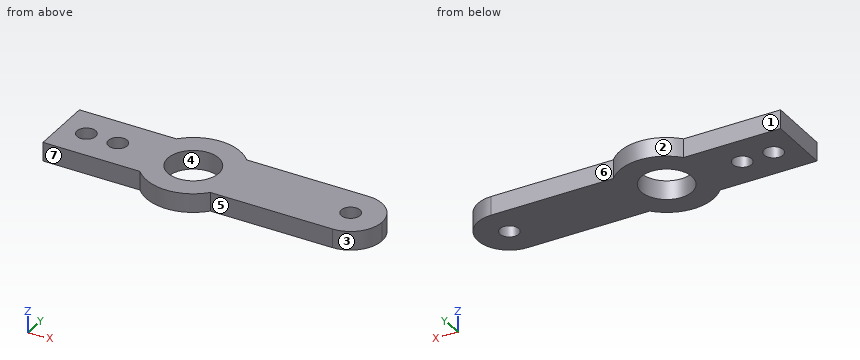
from build123d import *

# Parameters (mm, degrees)
F0_R     = 1.5
F0_R_2   = 4.05
F1_DEPTH = 3
F2_W     = 10
F2_H     = 3
F3_DEPTH = 9
F4_R     = 1.5
F5_DEPTH = 25
F6_R     = 4.99999


# Not quite as in the source:
# - a fillet or chamfer is up to 0.001 mm smaller than in the source, because OpenCascade refuses the exact size


with BuildPart() as f1:
    # F0 (on Top) → F1 (new body)
    with BuildSketch(Plane.XY):
        Polygon((21, -5), (21, 5), (5.5901699437, 5), (-5.5901699437, 5), (-21, 5), (-21, -5), (-5.5901699437, -5), (5.5901699437, -5), align=None)
        with Locations((-17, 0)):
            Circle(F0_R, mode=Mode.SUBTRACT)
        with Locations((-12, 0)):
            Circle(F0_R, mode=Mode.SUBTRACT)
        Circle(F0_R_2, mode=Mode.SUBTRACT)
        with BuildLine():
            Line((-5.5901699437, 5), (5.5901699437, 5))
            ThreePointArc((5.5901699437, 5), (0, 7.5), (-5.5901699437, 5))
        make_face()
        with BuildLine():
            ThreePointArc((-5.5901699437, -5), (0, -7.5), (5.5901699437, -5))
            Line((5.5901699437, -5), (-5.5901699437, -5))
        make_face()
    extrude(amount=F1_DEPTH)

    # F2 (on face) → F3 (join)
    with BuildSketch(Plane.YZ.offset(21)):
        with Locations((0, 1.5)):
            Rectangle(F2_W, F2_H)
    extrude(amount=F3_DEPTH)

    # F4 (on face) → F5 (cut)
    with BuildSketch(Plane(origin=(0, 0, 0), x_dir=(1, 0, 0), z_dir=(0, 0, -1))):
        with Locations((25, 0)):
            Circle(F4_R)
    extrude(amount=-F5_DEPTH, mode=Mode.SUBTRACT)

    # F6 (radius 5 in the source; OpenCascade refuses exactly that, so slightly less here)
    f6_edges = [f1.edges().sort_by_distance(p)[0] for p in [
        (30, -5, 1.5),
        (30, 5, 1.5),
    ]]
    fillet(f6_edges, radius=F6_R)


solid = f1.part
Check sheet for the modelled part. Datum: model origin and axes. Units: mm. Face numbers are marked on the shaded views. A direction names the side the tool comes from. Round coordinates to 2 decimals unless told otherwise and drop trailing zeros. Order: outer loops, then holes, each group sorted by start corner. A loop starts at its lowest first (then second) coordinate and runs counter-clockwise, first axis right, second up.
Q1. Cross-section at C-C, the plane z = 1.1. Give the number of separate pieces and of enclosed holes in the cut face, plus the area to 3 significant figures.
Filled sheet:
separate pieces: 1
enclosed holes: 4
area: 465 mm2
Q2. Set-up check for the marked faces 5, 6 and 7: record each of +Z, -Z, +X, -X, +Y, -Y from which the full face is reachable in a straight line by a thin tool's end or side.
Filled sheet:
face 5: +Z, -Z, +X, -Y
face 6: +Z, -Z, +X, +Y
face 7: +Z, -Z, -X, -Y
Q3. Draft check along X on the marked faces 1, 2, 3 and 4. Enter one of: pulls with the +X half, pulls with the -X half, needs draft (parallel to the pull), parting line crosses it, or undercut.
Filled sheet:
face 1: needs draft
face 2: parting line crosses it
face 3: pulls with the +X half
face 4: undercut
Q4. Cross-section at A-A, the plane x = 0. Enter the section's corners in (y, z), plus the area to 3 significant figures.
Filled sheet:
outline: (-7.5, 0) - (-4.05, 0) - (-4.05, 3) - (-7.5, 3) - close; (4.05, 0) - (7.5, 0) - (7.5, 3) - (4.05, 3) - close
area: 20.7 mm2
Q5. Cross-section at D-D, the plane x = 7.5. Enter the section's corners in (y, z).
Filled sheet:
outline: (-5, 0) - (5, 0) - (5, 3) - (-5, 3) - close
Q6. Cross-section at B-B, the plane y = 3.25. Enter the section's corners in (x, z).
Filled sheet:
outline: (-21, 0) - (-2.42, 0) - (-2.42, 3) - (-21, 3) - close; (2.42, 0) - (28.8, 0) - (28.8, 3) - (2.42, 3) - close
Q7. Depth check by flat-ended pin: P1, Ø3.5, axis at x = -12, y = 0, coming from the -Z side; P2, Ø0.9, axis at x = -11.5, z = 1.5, coming from the -Y side; P3, Ø1.5, axis at x = -9.5, z = 1.5, coming from the +Y side. Enter the tip coordinate at first touch or a pass-through.
Filled sheet:
P1: stops at z = 0
P2: stops at y = -5
P3: stops at y = 5
Q8. Scan lines: L1, parallel to Y at x = 25, z = 1.2; L2, parallel to Y at x = 0, z = 2.1; L3, parallel to X at y = -1, z = 2.3. Record each from-to range of solid material in increasing order.
Filled sheet:
L1: y = -5 to -1.5, 1.5 to 5
L2: y = -7.5 to -4.05, 4.05 to 7.5
L3: x = -21 to -18.12, -15.88 to -13.12, -10.88 to -3.92, 3.92 to 23.88, 26.12 to 29.9
